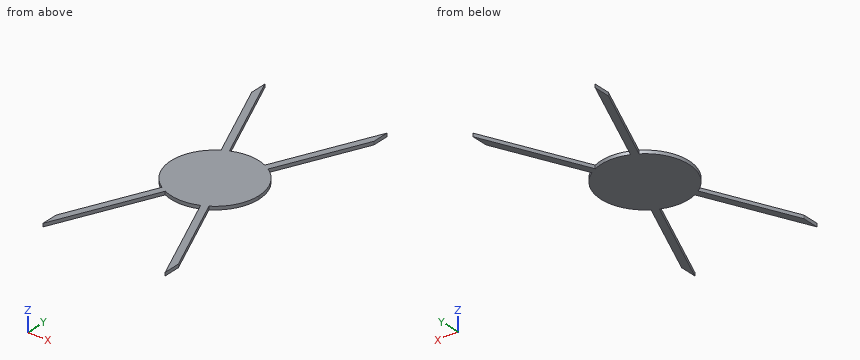
from build123d import *

# Parameters (mm, degrees)
F1_DEPTH = 3.175


with BuildPart() as f1:
    # F0 (on Top) → F1 (new body)
    with BuildSketch(Plane.XY):
        with BuildLine():
            ThreePointArc((81.351365, -168.93669), (95.692172, -153.651573), (100.901516, -133.34994))
            ThreePointArc((100.901516, -133.34994), (95.692172, -113.048307), (81.351365, -97.763191))
            ThreePointArc((81.351365, -97.763191), (78.599393, -96.157081), (75.733991, -94.763378))
            ThreePointArc((75.733991, -94.763378), (58.737516, -91.18594), (41.741042, -94.763378))
            ThreePointArc((41.741042, -94.763378), (38.87564, -96.157081), (36.123668, -97.763191))
            ThreePointArc((36.123668, -97.763191), (16.573516, -133.34994), (36.123668, -168.93669))
            ThreePointArc((36.123668, -168.93669), (38.87564, -170.542799), (41.741042, -171.936502))
            ThreePointArc((41.741042, -171.936502), (58.737516, -175.51394), (75.733991, -171.936502))
            ThreePointArc((75.733991, -171.936502), (78.599393, -170.542799), (81.351365, -168.93669))
        make_face()
        with BuildLine():
            ThreePointArc((75.733991, -94.763378), (78.599393, -96.157081), (81.351365, -97.763191))
            Line((81.351365, -97.763191), (117.475033, -15.752761))
            Line((117.475033, -15.752761), (117.475033, 0))
            Line((117.475033, 0), (75.733991, -94.763378))
        make_face()
        with BuildLine():
            Line((117.475033, -250.947119), (81.351365, -168.93669))
            ThreePointArc((81.351365, -168.93669), (78.599393, -170.542799), (75.733991, -171.936502))
            Line((75.733991, -171.936502), (117.475033, -266.69988))
            Line((117.475033, -266.69988), (117.475033, -250.947119))
        make_face()
        with BuildLine():
            ThreePointArc((36.123668, -97.763191), (38.87564, -96.157081), (41.741042, -94.763378))
            Line((41.741042, -94.763378), (0, 0))
            Line((0, 0), (0, -15.752761))
            Line((0, -15.752761), (36.123668, -97.763191))
        make_face()
        with BuildLine():
            Line((0, -266.69988), (41.741042, -171.936502))
            ThreePointArc((41.741042, -171.936502), (38.87564, -170.542799), (36.123668, -168.93669))
            Line((36.123668, -168.93669), (0, -250.947119))
            Line((0, -250.947119), (0, -266.69988))
        make_face()
    extrude(amount=-F1_DEPTH)


solid = f1.part
Read the model definition and answer for the solid it produces. Units are mm, in the model's axes. Give positions to 0.01 mm unless a question says otherwise; leave off trailing zeros. Loops run counter-clockwise (first coordinate to the right, second up) from the corner with the lowest first, then second, coordinate; pieces in that order, holes last. Notation, with made-up numbers: (-34.5, 89) -> (1.5, 89) arc R35 ccw to (1.5, 127) -> close; hole circle Ø7 at (54, -13). An arc over 180 degrees is marked (long way). Use a Markdown table: item, result.
Q1. Each of these flat-tipped pins is pushed along its axis until it touches: pin 1 (1 mm diameter, centred on y = -169.5, z = -1.5, fed in from +X); pin 2 (1 mm diameter, centred on y = -88.5, z = -1.5, fed in from +X). Where does it stop, or does it pass through?
Solved:
| item | result |
|---|---|
| pin 1 | stops at x = 81.82 |
| pin 2 | stops at x = 85.65 |
Q2. Section D-D, the plane x = 58.5 is taken. Determine the outline of the cut face in (y, z) (3 decimals).
Solved:
| item | result |
|---|---|
| outline | (-175.513, -3.175) -> (-91.187, -3.175) -> (-91.187, 0) -> (-175.513, 0) -> close |
Q3. Section A-A, the plane x = 26 is taken. Determine the outline of the cut face in (y, z) (3 decimals), then the cut area to 3 significant figures.
Solved:
| item | result |
|---|---|
| outline | (-207.673, -3.175) -> (-191.92, -3.175) -> (-191.92, 0) -> (-207.673, 0) -> close; (-159.922, -3.175) -> (-106.778, -3.175) -> (-106.778, 0) -> (-159.922, 0) -> close; (-74.78, -3.175) -> (-59.027, -3.175) -> (-59.027, 0) -> (-74.78, 0) -> close |
| area | 269 mm^2 |
Q4. Section B-B, the plane y = -69 is taken. Determine the outline of the cut face in (x, z) (3 decimals).
Solved:
| item | result |
|---|---|
| outline | (23.454, -3.175) -> (30.393, -3.175) -> (30.393, 0) -> (23.454, 0) -> close; (87.082, -3.175) -> (94.021, -3.175) -> (94.021, 0) -> (87.082, 0) -> close |
Q5. Section C-C, the plane z = -1.55 is taken. Determine the outline of the cut face in (x, y).
Solved:
| item | result |
|---|---|
| outline | (0, -266.7) -> (41.74, -171.94) arc R42.16 ccw to (75.73, -171.94) -> (117.48, -266.7) -> (117.48, -250.95) -> (81.35, -168.94) arc R42.16 ccw to (100.9, -133.35) arc R42.16 ccw to (81.35, -97.76) -> (117.48, -15.75) -> (117.48, 0) -> (75.73, -94.76) arc R42.16 ccw to (41.74, -94.76) -> (0, 0) -> (0, -15.75) -> (36.12, -97.76) arc R42.16 ccw to (36.12, -168.94) -> (0, -250.95) -> close |
Q6. Find the intervals of material crossed by line 1 along Y through (x, z) = (34, -1.45); line 2 along Y through (x, z) = (24, -1.65); line 3 along Y through (x, z) = (15, -2.9), in increasing order.
Solved:
| item | result |
|---|---|
| line 1 | y = -189.51 to -173.76, -167.49 to -99.21, -92.94 to -77.19 |
| line 2 | y = -212.21 to -196.46, -157.25 to -109.45, -70.24 to -54.49 |
| line 3 | y = -232.65 to -216.89, -49.81 to -34.05 |
